```python
from build123d import *

# Parameters (mm, degrees)
PAD_DEPTH       = 20
SKETCH004_R     = 2
POCKET002_DEPTH = 152.001
SKETCH005_R     = 2
POCKET003_DEPTH = 85.001


with BuildPart() as part:
    # Sketch → Pad (new body)
    with BuildSketch(Plane.XY):
        Polygon((-10, -42.5), (142, -42.5), (142, -30.5), (0, -30.5), (0, 30.5), (142, 30.5), (142, 42.5), (-10, 42.5), (-10, 38.5), (-17, 38.5), (-17, 33.5), (-10, 33.5), (-10, -33.5), (-17, -33.5), (-17, -38.5), (-10, -38.5), align=None)
    extrude(amount=PAD_DEPTH)

    # Sketch004 → Pocket002 (cut, through all)
    with BuildSketch(Plane(origin=(-10, 0, 0), x_dir=(0, -1, 0), z_dir=(-1, 0, 0))):
        with Locations((0, 10)):
            Circle(SKETCH004_R)
    extrude(amount=-POCKET002_DEPTH, mode=Mode.SUBTRACT)

    # Sketch005 → Pocket003 (cut, through all)
    with BuildSketch(Plane.XZ.offset(42.5)):
        with Locations((-5, 10)):
            Circle(SKETCH005_R)
        with Locations((132, 10)):
            Circle(SKETCH005_R)
    extrude(amount=-POCKET003_DEPTH, mode=Mode.SUBTRACT)


solid = part.part
```
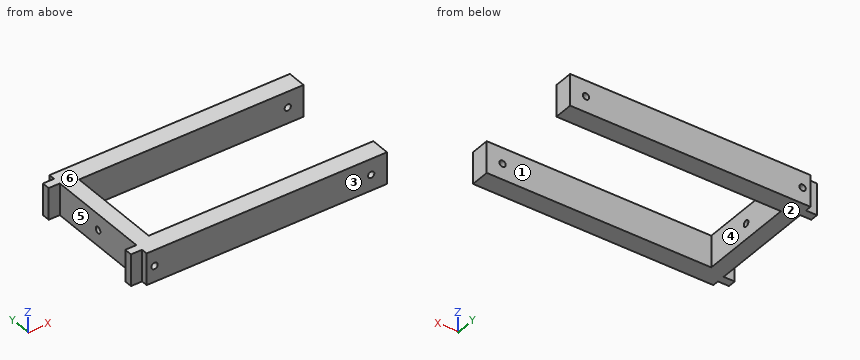
Input: part model. Units: mm. Frame: model coordinates. Face numbers are marked on the shaded views. A direction names the side the tool comes from. Coordinates: 2 decimals unless noted, no trailing zeros. Loops run counter-clockwise (first coordinate to the right, second up) from the corner with the lowest first, then second, coordinate; pieces in that order, holes last. Notation, with made-up numbers: M -19.5,-31 L 37.5,-31 A22 ccw 37.5,-20 Z; hole C -26.75,78 d3. An arc over 180 degrees is marked long. Use a Markdown table: item, result. Add a question column.
1) Set-up query: the marked faces 4, 5 and 6. Return all of +Z, -Z, +X, -X, +Y, -Y with unobstructed straight access to the full face (end or side cutting, diameter ignored); none if empty.
2) Line query: L1, parallel to Y at x = -7.25, z = 10; L2, parallel to Y at x = 38, z = 3.75; L3, parallel to X at y = 30, z = 10. Output: solid intervals per line, ascending. Write a range as from..to.
3) Section C-C, the plane x = 132. Return the cut outline in (y, z).
4) Section B-B, the plane y = 22.5. Return the cut outline in (x, z), plus the area to 3 significant figures.
5) Pin query (flat end, axial travel): P1, Ø6, axis at y = 5, z = 6, coming from the -X side; P2, Ø3.5, axis at x = -12.5, z = 14.5, coming from the -Y side; P3, Ø5.5, axis at x = -14.5, z = 14, coming from the +Y side. Return the tip coordinate at first contact, or that it passes through.
6) Section D-D, the plane z = 5.5. Return the cut outline in (x, y).
7) Section A-A, the plane x = 7.5. Return the cut outline in (y, z).
8) Draft query along Y for the marked faces 1, 2 and 3. Return one class per face: +Y half, -Y half, draft (parallel to the pull), parting line (faces both ways), or undercut.
Answer below:
| question | item | result |
|---|---|---|
| 1 | face 4 | +Z, -Z, +X |
| 1 | face 5 | +Z, -Z, -X |
| 1 | face 6 | +Z, +X, -X, +Y, -Y |
| 2 | L1 | -42.5..-2, 2..42.5 |
| 2 | L2 | -42.5..-30.5, 30.5..42.5 |
| 2 | L3 | -10..-7, -3..0 |
| 3 | outline | M -42.5,0 L -30.5,0 L -30.5,8 L -42.5,8 Z; M -42.5,12 L -30.5,12 L -30.5,20 L -42.5,20 Z; M 30.5,0 L 42.5,0 L 42.5,8 L 30.5,8 Z; M 30.5,12 L 42.5,12 L 42.5,20 L 30.5,20 Z |
| 4 | outline | M -10,0 L 0,0 L 0,20 L -10,20 Z; hole C -5,10 d4 |
| 4 | area | 187 mm2 |
| 5 | P1 | x = -10 |
| 5 | P2 | y = -38.5 |
| 5 | P3 | y = 38.5 |
| 6 | outline | M -17,-38.5 L -10,-38.5 L -10,-42.5 L 142,-42.5 L 142,-30.5 L 0,-30.5 L 0,30.5 L 142,30.5 L 142,42.5 L -10,42.5 L -10,38.5 L -17,38.5 L -17,33.5 L -10,33.5 L -10,-33.5 L -17,-33.5 Z |
| 7 | outline | M -42.5,0 L -30.5,0 L -30.5,20 L -42.5,20 Z; M 30.5,0 L 42.5,0 L 42.5,20 L 30.5,20 Z |
| 8 | face 1 | undercut |
| 8 | face 2 | draft |
| 8 | face 3 | -Y half |
